Build history of the part. All positions in model axes, mm. Round coordinates to 2 decimals unless told otherwise and drop trailing zeros. Order: outer loops, then holes, each group sorted by start corner. A loop starts at its lowest first (then second) coordinate and runs counter-clockwise, first axis right, second up. Notation, with made-up numbers: M -39.75,15.5 L -35.75,15.5 A8 ccw -35.75,26.5 Z; hole C -35,50 d6. An arc over 180 degrees is marked long. One line per question, with ' | ' between items. Start each with the question number.
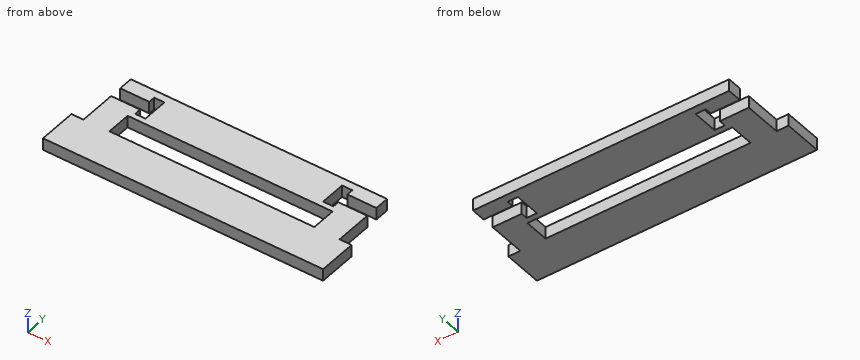
from build123d import *

# Parameters (mm, degrees)
SKETCH1_W           = 63.5
SKETCH1_H           = 25.4
SKETCH1_W_2         = 2.9718
SKETCH1_H_2         = 9.525
BOSS_EXTRUDE1_DEPTH = 2.9718
SKETCH2_W           = 50.8
SKETCH2_H           = 6.096
CUT_EXTRUDE1_DEPTH  = 3.9718
CUT_EXTRUDE2_DEPTH  = 3.9718


with BuildPart() as part:
    # Sketch1 → Boss-Extrude1 (new body)
    with BuildSketch(Plane.XY):
        Rectangle(SKETCH1_W, SKETCH1_H)
        with Locations((-33.2359, -7.9375)):
            Rectangle(SKETCH1_W_2, SKETCH1_H_2)
        with Locations((33.2359, -7.9375)):
            Rectangle(SKETCH1_W_2, SKETCH1_H_2)
    extrude(amount=BOSS_EXTRUDE1_DEPTH)

    # Sketch2 → Cut-Extrude1 (cut, through all)
    with BuildSketch(Plane.XY.offset(2.9718)):
        Rectangle(SKETCH2_W, SKETCH2_H)
    extrude(amount=-CUT_EXTRUDE1_DEPTH, mode=Mode.SUBTRACT)

    # Sketch3 → Cut-Extrude2 (cut, through all)
    with BuildSketch(Plane(origin=(0, 0, 0), x_dir=(-1, 0, 0), z_dir=(0, 0, -1))):
        Polygon((22.0218, 10.795), (22.0218, 4.445), (24.5618, 4.445), (24.5618, 6.096), (31.75, 6.096), (31.75, 9.144), (24.5618, 9.144), (24.5618, 10.795), align=None)
        Polygon((-31.75, 9.144), (-31.75, 6.096), (-24.5618, 6.096), (-24.5618, 4.445), (-22.0218, 4.445), (-22.0218, 10.795), (-24.5618, 10.795), (-24.5618, 9.144), align=None)
    extrude(amount=-CUT_EXTRUDE2_DEPTH, mode=Mode.SUBTRACT)


solid = part.part
Item 1: Wall check: line 1 along Y through (x, z) = (17.5, 1.9); line 2 along X through (y, z) = (1.5, 1.4); line 3 along Y through (x, z) = (29.5, 1.95). Give the ranges that are in metal, low to high. Write a range as [from, to].
Item 2: Cut at C-C on x = -21. Write the cut outline in (y, z).
Item 3: Cut at D-D on y = 8.25. Write the cut outline in (x, z), then the cut area to 3 significant figures.
Item 4: Cut at A-A on z = 2.2. Write the cut outline in (x, y) (3 decimals), then the cut area to 3 significant figures.
Item 5: Cut at B-B on y = -1. Write the cut outline in (x, z), then the cut area to 3 significant figures.
Item 6: Flat gauge pins, fed straight in: pin 1 (0.9 mm diameter, centred on y = 1.5, z = 1.5, fed in from +X); pin 2 (1.5 mm diameter, centred on y = 9.5, z = 0.5, fed in from -X); pin 3 (1.5 mm diameter, centred on y = 7.5, z = 1.5, fed in from -X). Where does each tip first touch, or does it go through?
Results found:
1) line 1: y = [-12.7, -3.05], [3.05, 12.7] | line 2: x = [-31.75, -25.4], [25.4, 31.75] | line 3: y = [-12.7, 6.1], [9.14, 12.7]
2) outline: M -12.7,0 L -3.05,0 L -3.05,2.97 L -12.7,2.97 Z; M 3.05,0 L 12.7,0 L 12.7,2.97 L 3.05,2.97 Z
3) outline: M -22.02,0 L 22.02,0 L 22.02,2.97 L -22.02,2.97 Z | area: 131 mm^2
4) outline: M -34.722,-12.7 L 34.722,-12.7 L 34.722,-3.175 L 31.75,-3.175 L 31.75,6.096 L 24.562,6.096 L 24.562,4.445 L 22.022,4.445 L 22.022,10.795 L 24.562,10.795 L 24.562,9.144 L 31.75,9.144 L 31.75,12.7 L -31.75,12.7 L -31.75,9.144 L -24.562,9.144 L -24.562,10.795 L -22.022,10.795 L -22.022,4.445 L -24.562,4.445 L -24.562,6.096 L -31.75,6.096 L -31.75,-3.175 L -34.722,-3.175 Z; hole M -25.4,-3.048 L 25.4,-3.048 L 25.4,3.048 L -25.4,3.048 Z | area: 1,280 mm^2
5) outline: M -31.75,0 L -25.4,0 L -25.4,2.97 L -31.75,2.97 Z; M 25.4,0 L 31.75,0 L 31.75,2.97 L 25.4,2.97 Z | area: 37.7 mm^2
6) pin 1: stops at x = 31.75 | pin 2: stops at x = -31.75 | pin 3: stops at x = -22.02
